The model under review builds one solid part; all positions refer to its coordinate system, in mm. Face numbers are marked on the shaded views. A direction names the side the tool comes from. Round coordinates to 2 decimals unless told otherwise and drop trailing zeros. Write each loop counter-clockwise with the first axis right and the second up, starting at its lowest first coordinate (ties: lowest second). Pieces come first, ordered by that corner, then holes. Notation, with made-up numbers: (3.5, 53) -> (12.5, 53) arc R13 ccw to (12.5, 73) -> close; hole circle Ø3 at (63.25, 50.25). An arc over 180 degrees is marked (long way). Answer as a JSON object with one key per item and string values. Group by question number.
1) To check wall thickness, follow probe 1 along Y at (x, z) = (21, 3.05); probe 2 along Z at (x, y) = (54.5, 10.25); probe 3 along X at (y, z) = (2.75, 36). State the ranges of each line that lie inside material, in increasing order. Write a range as [from, to].
2) Insertion check: pin 1 Ø7.5 at (y, z) = (9, 15) entering from +X; pin 2 Ø4 at (x, y) = (90.5, 7.5) entering from +Z. Each pin has a flat end and moves straight along its axis. Give the tip position at first contact, or say it passes through.
3) Machinability: for the marked faces 1 and 2, which of the approach directions +Z, -Z, +X, -X, +Y, -Y give a long, thin tool a straight path to every point of the face, cutting with its end or side? Answer none if there is none.
4) We need section C-C, the plane z = 14. Write out the cut boundary in (x, y).
5) We need section D-D, the plane z = 23. Write out the cut boundary in (x, y), then the cut area to 3 significant figures.
6) We need section A-A, the plane x = 90.5. Write out the cut boundary in (y, z).
7) We need section B-B, the plane y = 3.25. Write out the cut boundary in (x, z), then the cut area to 3 significant figures.
from build123d import *

# Parameters (mm, degrees)
SKETCH1_W             = 140
SKETCH1_H             = 15
BOSS_EXTRUDE1_DEPTH   = 4
M3X0_5_TAPPED_HOLE1_D = 2.5
SKETCH6_W             = 40
SKETCH6_H             = 15
BOSS_EXTRUDE2_DEPTH   = 4
FILLET1_R             = 2
F_4_0MM_DOWEL_HOLE1_D = 4.2


with BuildPart() as part:
    # Sketch1 → Boss-Extrude1 (new body)
    with BuildSketch(Plane.XY):
        with Locations((70, 7.5)):
            Rectangle(SKETCH1_W, SKETCH1_H)
    extrude(amount=BOSS_EXTRUDE1_DEPTH)

    # M3x0.5 Tapped Hole1 (through all)
    with Locations(Plane(origin=(0, 0, 0), x_dir=(-1, 0, 0), z_dir=(0, 0, -1))):
        with Locations((-130, 7.5), (-116, 7.5), (-90.5, 7.5), (-60.5, 7.5), (-46.5, 7.5), (-21, 7.5)):
            Hole(M3X0_5_TAPPED_HOLE1_D / 2)

    # Sketch6 → Boss-Extrude2 (add)
    with BuildSketch(Plane.ZY):
        with Locations((20, 7.5)):
            Rectangle(SKETCH6_W, SKETCH6_H)
    extrude(amount=BOSS_EXTRUDE2_DEPTH)

    # Fillet1
    fillet1_edges = [part.edges().sort_by_distance(p)[0] for p in [
        (0, 7.5, 4),
        (-4, 7.5, 0),
    ]]
    fillet(fillet1_edges, radius=FILLET1_R)

    # Ø4.0mm Dowel Hole1 (through all)
    with Locations(Plane.ZY.offset(4)):
        with Locations((34, 7.5), (14, 7.5)):
            Hole(F_4_0MM_DOWEL_HOLE1_D / 2)


solid = part.part
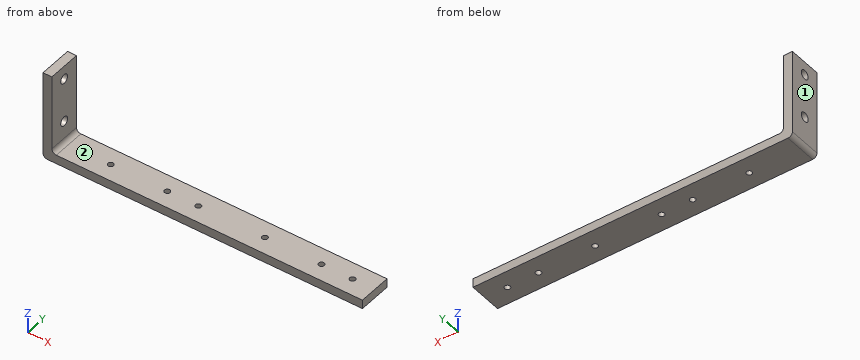
Here are the results:
{
 "1": {"probe 1": "y = [0, 6.25], [8.75, 15]", "probe 2": "z = [0, 4]", "probe 3": "x = [-4, 0]"},
 "2": {"pin 1": "stops at x = 0", "pin 2": "stops at z = 4"},
 "3": {"face 1": "+Z, -Z, -X, +Y, -Y", "face 2": "+Z, +X, +Y, -Y"},
 "4": {"outline": "(-4, 0) -> (0, 0) -> (0, 5.4) -> (-4, 5.4) -> close; (-4, 9.6) -> (0, 9.6) -> (0, 15) -> (-4, 15) -> close"},
 "5": {"outline": "(-4, 0) -> (0, 0) -> (0, 15) -> (-4, 15) -> close", "area": "60.0 mm^2"},
 "6": {"outline": "(0, 0) -> (6.25, 0) -> (6.25, 4) -> (0, 4) -> close; (8.75, 0) -> (15, 0) -> (15, 4) -> (8.75, 4) -> close"},
 "7": {"outline": "(-4, 2) arc R2 ccw to (-2, 0) -> (140, 0) -> (140, 4) -> (2, 4) arc R2 cw to (0, 6) -> (0, 40) -> (-4, 40) -> close", "area": "720 mm^2"}
}
